```python
from build123d import *

# Parameters (mm, degrees)
F0_W     = 50.08647
F0_H     = 130
F1_DEPTH = 5
F2_R     = 3
F2_R_2   = 2.25
F3_DEPTH = 25
F4_DEPTH = 4
F5_W     = 3
F5_H     = 130
F6_DEPTH = 3


with BuildPart() as f1:
    # F0 (on Top) → F1 (new body)
    with BuildSketch(Plane.XY):
        with Locations((-10.767537, -34.325769)):
            Rectangle(F0_W, F0_H)
    extrude(amount=F1_DEPTH)

    # F2 (on face) → F3 (cut)
    with BuildSketch(Plane.XY.offset(5)):
        with Locations((-10.980115, -89.325769)):
            Circle(F2_R)
        with Locations((8.176511, 23.25341)):
            Circle(F2_R_2)
        with Locations((-29.718949, 23.25341)):
            Circle(F2_R_2)
    extrude(amount=-F3_DEPTH, mode=Mode.SUBTRACT)

    # F2 (on face) → F4 (cut)
    with BuildSketch(Plane.XY.offset(5)):
        Polygon((10.226105, 26.80341), (6.126918, 26.80341), (4.077324, 23.25341), (6.126918, 19.70341), (10.226105, 19.70341), (12.275698, 23.25341), align=None)
        with Locations((8.176511, 23.25341)):
            Circle(F2_R_2, mode=Mode.SUBTRACT)
        Polygon((-31.977558, 26.674231), (-33.810772, 23.007808), (-31.552163, 19.586987), (-27.46034, 19.832589), (-25.627126, 23.499012), (-27.885736, 26.919834), align=None)
        with Locations((-29.718949, 23.25341)):
            Circle(F2_R_2, mode=Mode.SUBTRACT)
        Polygon((-10.428065, -83.288779), (-15.932276, -85.829184), (-16.484327, -91.866174), (-11.532166, -95.362758), (-6.027954, -92.822353), (-5.475904, -86.785364), align=None)
        with Locations((-10.980115, -89.325769)):
            Circle(F2_R, mode=Mode.SUBTRACT)
    extrude(amount=-F4_DEPTH, mode=Mode.SUBTRACT)

    # F5 (on face) → F6 (join)
    with BuildSketch(Plane.XY.offset(5)):
        with Locations((1.775698, -34.325769)):
            Rectangle(F5_W, F5_H)
        with Locations((-23.310772, -34.325769)):
            Rectangle(F5_W, F5_H)
    extrude(amount=F6_DEPTH)


solid = f1.part
```
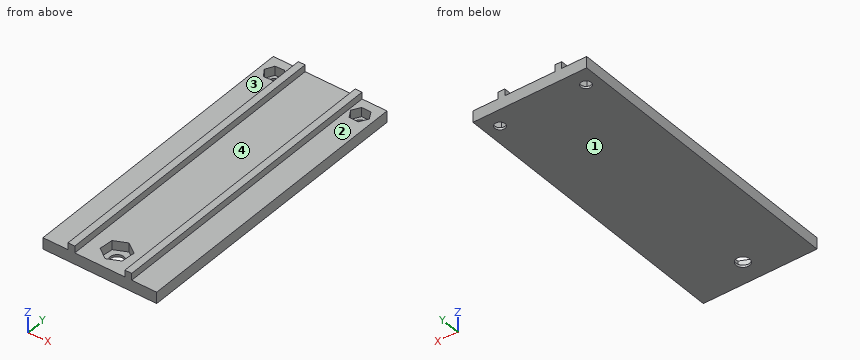
Check sheet for the modelled part. Datum: model origin and axes. Units: mm. Face numbers are marked on the shaded views. A direction names the side the tool comes from. Give positions to 0.01 mm unless a question says otherwise; leave off trailing zeros. Order: outer loops, then holes, each group sorted by start corner. A loop starts at its lowest first (then second) coordinate and runs counter-clockwise, first axis right, second up. Notation, with made-up numbers: (-17, 56) -> (-7, 56) arc R18 ccw to (-7, 88) -> close; hole circle Ø1 at (81, -15.5). An arc over 180 degrees is marked (long way). Return JSON: item names as keys, results as strings.
1. Cross-section at C-C, the plane x = -18.5. Record the cut outline in (y, z).
From the geometry:
{"outline": "(-99.33, 0) -> (30.67, 0) -> (30.67, 5) -> (-99.33, 5) -> close"}
2. Cross-section at A-A, the plane z = 2.5. Record the cut outline in (x, y).
From the geometry:
{"outline": "(-35.81, -99.33) -> (14.28, -99.33) -> (14.28, 30.67) -> (-35.81, 30.67) -> close; hole (-33.81, 23.01) -> (-31.55, 19.59) -> (-27.46, 19.83) -> (-25.63, 23.5) -> (-27.89, 26.92) -> (-31.98, 26.67) -> close; hole (-16.48, -91.87) -> (-11.53, -95.36) -> (-6.03, -92.82) -> (-5.48, -86.79) -> (-10.43, -83.29) -> (-15.93, -85.83) -> close; hole (4.08, 23.25) -> (6.13, 19.7) -> (10.23, 19.7) -> (12.28, 23.25) -> (10.23, 26.8) -> (6.13, 26.8) -> close"}
3. Mould release check, pull along X, two halves, no side actions. Record for the marked faces 3 and 4: +X half, -X half, draft (parallel to the pull), parting line (faces both ways), or undercut.
From the geometry:
{"face 3": "draft", "face 4": "undercut"}
4. Set-up check for the marked faces 1 and 2: record each of +Z, -Z, +X, -X, +Y, -Y from which the full face is reachable in a straight line by a thin tool's end or side.
From the geometry:
{"face 1": "-Z, +X, -X, +Y, -Y", "face 2": "+Z, +X, +Y, -Y"}
5. Go/stop test with flat-tipped pins: P1, Ø3.5, axis at x = -32, y = -12, coming from the +Z side; P2, Ø5, axis at x = -29.72, y = 23.25, coming from the +Z side; P3, Ø1.5, axis at y = -38, z = 6, coming from the +X side; P4, Ø4, axis at x = 8.18, y = 23.25, coming from the -Z side. Record where each tip stops, or that it passes through.
From the geometry:
{"P1": "z = 5", "P2": "z = 1", "P3": "x = 3.28", "P4": "through"}
6. Material ranges on probe 1 along X at (y, z) = (-63, 7); probe 2 along Z at (x, y) = (6, -7); probe 3 along Y at (x, z) = (-8.5, 2.25), recorded low to high. Write a range as [from, to].
From the geometry:
{"probe 1": "[-24.81, -21.81], [0.28, 3.28]", "probe 2": "[0, 5]", "probe 3": "[-99.33, -93.96], [-84.65, 30.67]"}
7. Cross-section at B-B, the plane y = 12.5. Record the cut outline in (x, z), plus the area to 3 significant figures.
From the geometry:
{"outline": "(-35.81, 0) -> (14.28, 0) -> (14.28, 5) -> (3.28, 5) -> (3.28, 8) -> (0.28, 8) -> (0.28, 5) -> (-21.81, 5) -> (-21.81, 8) -> (-24.81, 8) -> (-24.81, 5) -> (-35.81, 5) -> close", "area": "268 mm^2"}
